from build123d import *

# Parameters (mm, degrees)
F0_R     = 38.1
F0_R_2   = 25.4
F1_DEPTH = 100
F2_R     = 56.791086
F2_R_2   = 25.414512
F3_DEPTH = 25
F4_R     = 2
F5_R     = 2


with BuildPart() as f1:
    # F0 (on Front) → F1 (new body)
    with BuildSketch(Plane.XZ):
        with Locations((0, 36.864621)):
            Circle(F0_R)
        with Locations((0, 36.864621)):
            Circle(F0_R_2, mode=Mode.SUBTRACT)
    extrude(amount=F1_DEPTH)

    # F2 (on face) → F3 (join)
    with BuildSketch(Plane.XZ.offset(100)):
        with Locations((0, 36.864621)):
            Circle(F2_R)
        with Locations((0, 36.864621)):
            Circle(F2_R_2, mode=Mode.SUBTRACT)
    extrude(amount=-F3_DEPTH)

    # F4
    f4_edges = [f1.edges().sort_by_distance(p)[0] for p in [
        (-38.1, 0, 36.864621),
    ]]
    fillet(f4_edges, radius=F4_R)

    # F5
    f5_edges = [f1.edges().sort_by_distance(p)[0] for p in [
        (-25.4, -100, 36.864621),
    ]]
    fillet(f5_edges, radius=F5_R)


solid = f1.part
The model under review builds one solid part; all positions refer to its coordinate system, in mm. A direction names the side the tool comes from. Round coordinates to 2 decimals unless told otherwise and drop trailing zeros. Write each loop counter-clockwise with the first axis right and the second up, starting at its lowest first coordinate (ties: lowest second). Pieces come first, ordered by that corner, then holes. Notation, with made-up numbers: (-32.5, 29.5) - (-22.5, 29.5) arc R13 cw to (-22.5, 40.5) - close; hole circle Ø10 at (-24.5, 55.25). An arc over 180 degrees is marked (long way). One line per item, written item: value. Start each with the question number.
1. Consider section A-A on x = 0. Write out the cut boundary in (y, z), and give its area (3 significant figures).
2. The part is to be moulded in two halves that separate along Z. For faces 3 (the face through (-41.9, -87.7, 75.2)), 4 (the face through (37, -75, 25)), 5 (the face through (-3.31, -48.31, 62.05)), say which applies: released by +Z, released by -Z, zero draft, split by the parting line, or undercut.
3. Clearance check with flat-ended pins moving along their axes: P1, Ø3, axis at x = 23.5, z = -1, coming from the +Y side; P2, Ø6, axis at y = -38, z = 57.5, coming from the -X side; P3, Ø6, axis at y = -47.5, z = 39.5, coming from the +X side. State where each tip first meets the part, or that it passes through.
4. Consider section B-B on y = -65. Write out the cut boundary in (x, z), and give its area (3 significant figures).
5. Consider section C-C on z = -9.5. Write out the cut boundary in (x, y), and give its area (3 significant figures).
6. Machinability: for faces 1 (the face through (-25, 0, 29)), 2 (the face through (-8.26, -37.99, -0.33)), which of the approach directions +Z, -Z, +X, -X, +Y, -Y give a long, thin tool a straight path to every point of the face, cutting with its end or side? Answer none if there is none.
7. To check wall thickness, follow L1, parallel to Z at x = 0, y = -43; L2, parallel to Z at x = 1, y = -94; L3, parallel to X at y = -74, z = 56. State the ranges of each line that lie inside material, in increasing order. Write a range as from..to.
Checks:
1. outline: (-100, -19.93) - (-75, -19.93) - (-75, -1.24) - (-2, -1.24) arc R2 ccw to (0, 0.76) - (0, 11.46) - (-98, 11.46) arc R2 ccw to (-100, 9.46) - close; (-100, 64.26) arc R2 ccw to (-98, 62.26) - (0, 62.26) - (0, 72.96) arc R2 ccw to (-2, 74.96) - (-75, 74.96) - (-75, 93.66) - (-100, 93.66) - close
1. area: 3,470 mm^2
2. face 3: split by the parting line
2. face 4: zero draft
2. face 5: undercut
3. P1: stops at y = -75
3. P2: stops at x = -33.77
3. P3: stops at x = 38.1
4. outline: circle Ø76.2 at (0, 36.86); hole circle Ø50.8 at (0, 36.86)
4. area: 2,530 mm^2
5. outline: (-32.8, -100) - (32.8, -100) - (32.8, -75) - (-32.8, -75) - close
5. area: 1,640 mm^2
6. face 1: +Z, -Z, +X, -X, +Y
6. face 2: +Y
7. L1: z = -1.24..11.46, 62.26..74.96
7. L2: z = -19.92..11.48, 62.24..93.65
7. L3: x = -32.95..-16.7, 16.7..32.95
